Here's how the part is built. I have some questions about the finished solid (model axes, mm). A direction names the side the tool comes from. Give positions to 0.01 mm unless a question says otherwise; leave off trailing zeros. Loops run counter-clockwise (first coordinate to the right, second up) from the corner with the lowest first, then second, coordinate; pieces in that order, holes last. Notation, with made-up numbers: (70, 81) - (104, 81) arc R10 cw to (104, 89) - close; hole circle Ø5 at (-33.5, -32). An arc over 180 degrees is marked (long way). One line per item, written item: value. Start each with the question number.
```python
from build123d import *

# Parameters (mm, degrees)
SKETCH1_R                        = 6.35
BUSHINGSPROCKETSPACE_DEPTH       = 31.75
SKETCH2_R                        = 10.033
BOSS_EXTRUDE2_DEPTH              = 64.3509
SKETCH3_R                        = 6.35
BOSS_EXTRUDE3_DEPTH              = 12.7
F_10_24_TAPPED_HOLE2_D           = 3.7973
F_10_24_TAPPED_HOLE2_DEPTH       = 10.16
F_10_24_TAPPED_HOLE2_CSINK_D     = 5.0673
F_10_24_TAPPED_HOLE2_CSINK_ANGLE = 90
F_10_24_TAPPED_HOLE2_TIP         = 1.140824014


with BuildPart() as part:
    # Sketch1 → BushingSprocketSpace (new body)
    with BuildSketch(Plane(origin=(0, 0, 0), x_dir=(1, 0, 0), z_dir=(0, 1, 0))):
        Circle(SKETCH1_R)
    extrude(amount=BUSHINGSPROCKETSPACE_DEPTH)

    # Sketch2 → Boss-Extrude2 (add)
    with BuildSketch(Plane(origin=(0, 31.75, 0), x_dir=(1, 0, 0), z_dir=(0, 1, 0))):
        Circle(SKETCH2_R)
    extrude(amount=BOSS_EXTRUDE2_DEPTH)

    # Sketch3 → Boss-Extrude3 (add)
    with BuildSketch(Plane(origin=(0, 96.1009, 0), x_dir=(1, 0, 0), z_dir=(0, 1, 0))):
        Circle(SKETCH3_R)
    extrude(amount=BOSS_EXTRUDE3_DEPTH)

    # #10-24 Tapped Hole2
    with Locations(Plane(origin=(0, 64.25184, -10.033), x_dir=(-1, 0, 0), z_dir=(0, 0, -1))):
        with Locations((0, 0)):
            CounterSinkHole(F_10_24_TAPPED_HOLE2_D / 2, F_10_24_TAPPED_HOLE2_CSINK_D / 2, depth=F_10_24_TAPPED_HOLE2_DEPTH, counter_sink_angle=F_10_24_TAPPED_HOLE2_CSINK_ANGLE)
            with Locations((0, 0, -(F_10_24_TAPPED_HOLE2_DEPTH + F_10_24_TAPPED_HOLE2_TIP / 2))):  # 118° drill point
                Cone(0, F_10_24_TAPPED_HOLE2_D / 2, F_10_24_TAPPED_HOLE2_TIP, mode=Mode.SUBTRACT)


solid = part.part
```
(1) If we section it at B-B on x = -3.25: List the corners of the cut face in (y, z) for me, plus the area to 3 significant figures.
(2) If we section it at A-A on z = -4: List the corners of the cut face in (x, y) for me, plus the area to 3 significant figures.
(3) For faces 4 (the face through (-0.41, 62.4, -4.57)), 5 (the face through (-1.38, 102.36, 6.2)), 6 (the face through (-1.38, 15.65, 6.2)), which set-ups out of +Z, -Z, +X, -X, +Y, -Y let a thin tool reach every point of the face, with its end or its side?
(4) If we mould it in two halves opening along X, with no side actions, what happens to faces 1 (the face through (0, 96.101, 7)), 2 (the face through (-2.175, 63.475, 9.794)), 3 (the face through (-0.18, 64.53, 1.07))? For each: pulls with the +X half, pulls with the -X half, needs draft (parallel to the pull), parting line crosses it, or undercut.
(5) Will these pins go through, and if not, where does the flat tip stop? pin 1 (1.5 mm diameter, centred on y = 26.5, z = 4, fed in from -X); pin 2 (2 mm diameter, centred on x = 4.5, y = 65, fed in from +Z); pin 3 (3 mm diameter, centred on y = 75.5, z = -6.5, fed in from +X).
(6) If we section it at C-C on y = 45.5: List the corners of the cut face in (x, z) for me.
(7) Please list where these lines run through material, in increasing order: probe 1 along Y at (x, z) = (0, -4); probe 2 along Y at (x, z) = (0.5, -8.25); probe 3 along Z at (x, y) = (0.25, 32). Write a range as from..to.
(8) If we section it at D-D on z = 4.5: List the corners of the cut face in (x, y) for me.
Found:
1. outline: (0, -5.46) - (31.75, -5.46) - (31.75, -9.49) - (96.1, -9.49) - (96.1, -5.46) - (108.8, -5.46) - (108.8, 5.46) - (96.1, 5.46) - (96.1, 9.49) - (31.75, 9.49) - (31.75, 5.46) - (0, 5.46) - close
1. area: 1,710 mm^2
2. outline: (-9.2, 31.75) - (-4.93, 31.75) - (-4.93, 0) - (4.93, 0) - (4.93, 31.75) - (9.2, 31.75) - (9.2, 96.1) - (4.93, 96.1) - (4.93, 108.8) - (-4.93, 108.8) - (-4.93, 96.1) - (-9.2, 96.1) - close; hole circle Ø3.8 at (0, 64.25)
2. area: 1,610 mm^2
3. face 4: -Z
3. face 5: +Y
3. face 6: -Y
4. face 1: needs draft
4. face 2: parting line crosses it
4. face 3: undercut
5. pin 1: x = -5.46
5. pin 2: z = 9.4
5. pin 3: x = 8.7
6. outline: circle Ø20.07 at (0, 0)
7. probe 1: 0..62.35, 66.15..108.8
7. probe 2: 31.75..62.42, 66.08..96.1
7. probe 3: -10.03..10.03
8. outline: (-8.97, 31.75) - (-4.48, 31.75) - (-4.48, 0) - (4.48, 0) - (4.48, 31.75) - (8.97, 31.75) - (8.97, 96.1) - (4.48, 96.1) - (4.48, 108.8) - (-4.48, 108.8) - (-4.48, 96.1) - (-8.97, 96.1) - close
